Study the drawing (mm; zero at the part's minimum x, y, z) and answer. A direction names the side the tool comes from. Round coordinates to 2 decimals unless told otherwise and drop trailing zeros. Write each loop counter-clockwise with the first axis right and the second up, starting at its lowest first coordinate (ties: lowest second). Pieces come first, ordered by that corner, then holes. Notation, with made-up numbers: (74, 56.5) -> (115, 56.5) arc R16 cw to (115, 84.5) -> close; hole circle Ø6 at (48.5, 7.5). An arc over 180 degrees is marked (long way). Return JSON: item names as keys, results as strings.
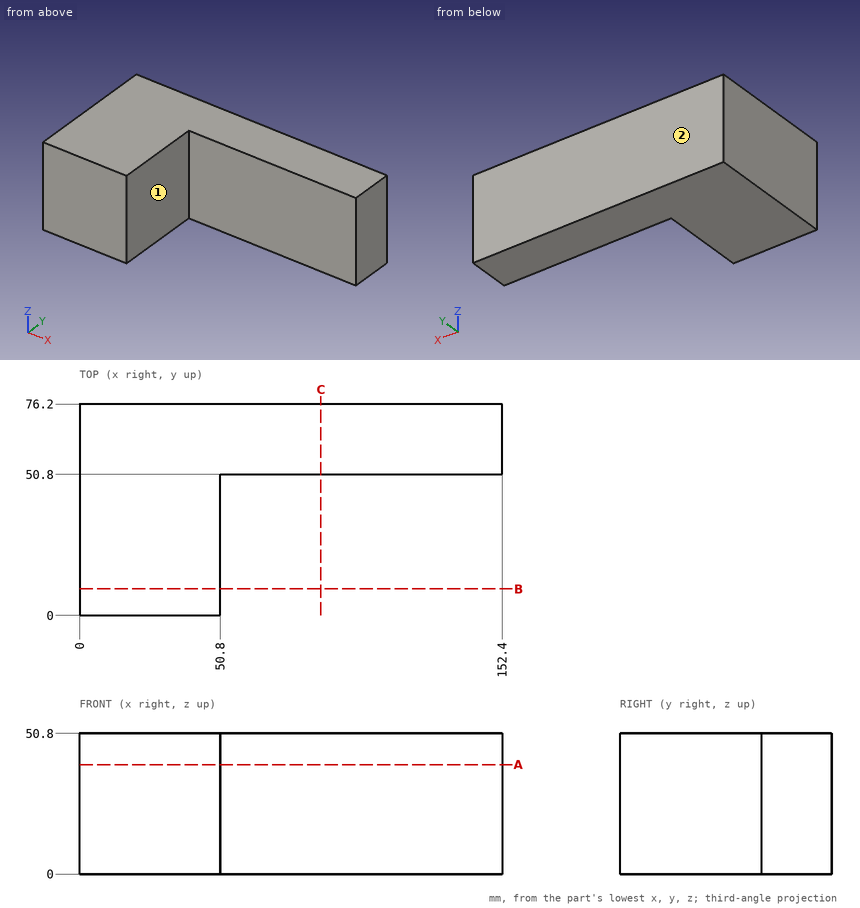
Item 1: Flat-ended cylindrical pins translate along their axes: pin 1 (12 mm diameter, centred on x = 111.5, z = 23, fed in from -Y); pin 2 (12 mm diameter, centred on x = 132, y = 57.5, fed in from -Z). Find the tip coordinate at first contact, or state that the pin passes through.
Worked answers:
{"pin 1": "stops at y = 50.8", "pin 2": "stops at z = 0"}
Item 2: Straight lines are drawn through the part: L1, parallel to Y at x = 146.5, z = 30; L2, parallel to X at y = 44, z = 24.5. For each, find the intervals that lie inside material, in ascending order. Write a range as [from, to].
Worked answers:
{"L1": "y = [50.8, 76.2]", "L2": "x = [0, 50.8]"}
Item 3: Section C-C (x = 87) is taken. Give the vertices of the cut face in (y, z).
Worked answers:
{"outline": "(50.8, 0) -> (76.2, 0) -> (76.2, 50.8) -> (50.8, 50.8) -> close"}
Item 4: A tool of negligible diameter and unlimited length cuts with its end or side. For the marked faces 1 and 2, from which of +Z, -Z, +X, -X, +Y, -Y can it reach the whole face along a straight path? Write none if from no direction.
Worked answers:
{"face 1": "+Z, -Z, +X, -Y", "face 2": "+Z, -Z, +X, -X, +Y"}
Item 5: Section A-A (z = 39.5) is taken. Give the vertices of the cut face in (x, y).
Worked answers:
{"outline": "(0, 0) -> (50.8, 0) -> (50.8, 50.8) -> (152.4, 50.8) -> (152.4, 76.2) -> (0, 76.2) -> close"}
Item 6: Section B-B (y = 9.5) is taken. Give the vertices of the cut face in (x, z).
Worked answers:
{"outline": "(0, 0) -> (50.8, 0) -> (50.8, 50.8) -> (0, 50.8) -> close"}
